from build123d import *

# Parameters (mm, degrees)
F0_W     = 48
F0_H     = 30
F1_DEPTH = 34
F2_R     = 14
F2_R_2   = 11
F3_DEPTH = 30
F4_DEPTH = 23
F6_D     = 1
F6_DEPTH = 12
F6_TIP   = 0.3004303095


with BuildPart() as f1:
    # F0 (on Front) → F1 (new body)
    with BuildSketch(Plane.XZ):
        Rectangle(F0_W, F0_H)
    extrude(amount=F1_DEPTH)

    # F2 (on face) → F3 (join)
    with BuildSketch(Plane.XZ.offset(34)):
        Circle(F2_R)
        Circle(F2_R_2, mode=Mode.SUBTRACT)
    extrude(amount=F3_DEPTH)

    # F4 (add): a face of the model
    f4_faces = [f1.faces().sort_by_distance(p)[0] for p in [
        (0, -34, 0),
    ]]
    extrude(f4_faces, amount=F4_DEPTH)

    # F6
    with Locations(Plane.XZ.offset(64)):
        with Locations((0, 12.5), (-10.8253175473, 6.25), (-10.8253175473, -6.25), (0, -12.5), (10.8253175473, -6.25), (10.8253175473, 6.25)):
            Hole(F6_D / 2, depth=F6_DEPTH)
            with Locations((0, 0, -(F6_DEPTH + F6_TIP / 2))):  # 118° drill point
                Cone(0, F6_D / 2, F6_TIP, mode=Mode.SUBTRACT)


solid = f1.part
Here's how the part is built. I have some questions about the finished solid (model axes, mm). A direction names the side the tool comes from. Round coordinates to 2 decimals unless told otherwise and drop trailing zeros. Loops run counter-clockwise (first coordinate to the right, second up) from the corner with the lowest first, then second, coordinate; pieces in that order, holes last. Notation, with made-up numbers: (43, 18.5) -> (66, 18.5) arc R32 cw to (66, 50.5) -> close; hole circle Ø7 at (54, 37.25). An arc over 180 degrees is marked (long way). Write each question's results on one line, items separated by ' | '.
(1) We'd pull the mould along X, two halves only. Please class faces 1 (the face through (0, 0, 0)), 2 (the face through (-2.38, -60.45, -10.74)), 3 (the face through (12.932, -48.79, -5.362)): released by +X, released by -X, zero draft, split by the parting line, or undercut.
Worked answers:
face 1: zero draft | face 2: undercut | face 3: split by the parting line
(2) If we section it at B-B, the plane z = 0: List the corners of the cut face in (x, y) for me.
Worked answers:
outline: (-24, -34) -> (-14, -34) -> (-14, -64) -> (-11, -64) -> (-11, -57) -> (11, -57) -> (11, -64) -> (14, -64) -> (14, -34) -> (24, -34) -> (24, 0) -> (-24, 0) -> close
(3) For faces 4 (the face through (-6, -34, -13)), 5 (the face through (24, -17, 0)), which set-ups out of +Z, -Z, +X, -X, +Y, -Y let a thin tool reach every point of the face, with its end or its side?
Worked answers:
face 4: -Y | face 5: +Z, -Z, +X, +Y, -Y
(4) For P1, Ø2, axis at x = 7.5, z = -3, coming from the -Y side; P2, Ø5, axis at x = -17.5, z = -3.5, coming from the -Y side; P3, Ø5, axis at y = -53, z = -1, coming from the -X side, each with a flat end and sliding along its axis, tell me the tip position at first contact or that it passes through.
Worked answers:
P1: y = -57 | P2: y = -34 | P3: x = -14
(5) If we section it at D-D, the plane y = -50: List the corners of the cut face in (x, z) for me.
Worked answers:
outline: circle Ø28 at (0, 0)
(6) If we section it at C-C, the plane x = -15: List the corners of the cut face in (y, z) for me.
Worked answers:
outline: (-34, -15) -> (0, -15) -> (0, 15) -> (-34, 15) -> close
(7) If I drill on L1, parallel to Z at x = 0, y = -56.5; L2, parallel to Z at x = 0, y = -59.25; L3, parallel to X at y = -61, z = -6.25, over which ranges is the centre line in solid material (lowest first)?
Worked answers:
L1: -14 to -13, -12 to 12, 13 to 14 | L2: -14 to -13, -12 to -11, 11 to 12, 13 to 14 | L3: -12.53 to -11.33, -10.33 to -9.05, 9.05 to 10.33, 11.33 to 12.53
(8) If we section it at A-A, the plane y = -58.5: List the corners of the cut face in (x, z) for me, then the cut area to 3 significant figures.
Worked answers:
outline: circle Ø28 at (0, 0); hole circle Ø1 at (-10.83, -6.25); hole circle Ø1 at (-10.83, 6.25); hole circle Ø22 at (0, 0); hole circle Ø1 at (0, -12.5); hole circle Ø1 at (0, 12.5); hole circle Ø1 at (10.83, -6.25); hole circle Ø1 at (10.83, 6.25) | area: 231 mm2
